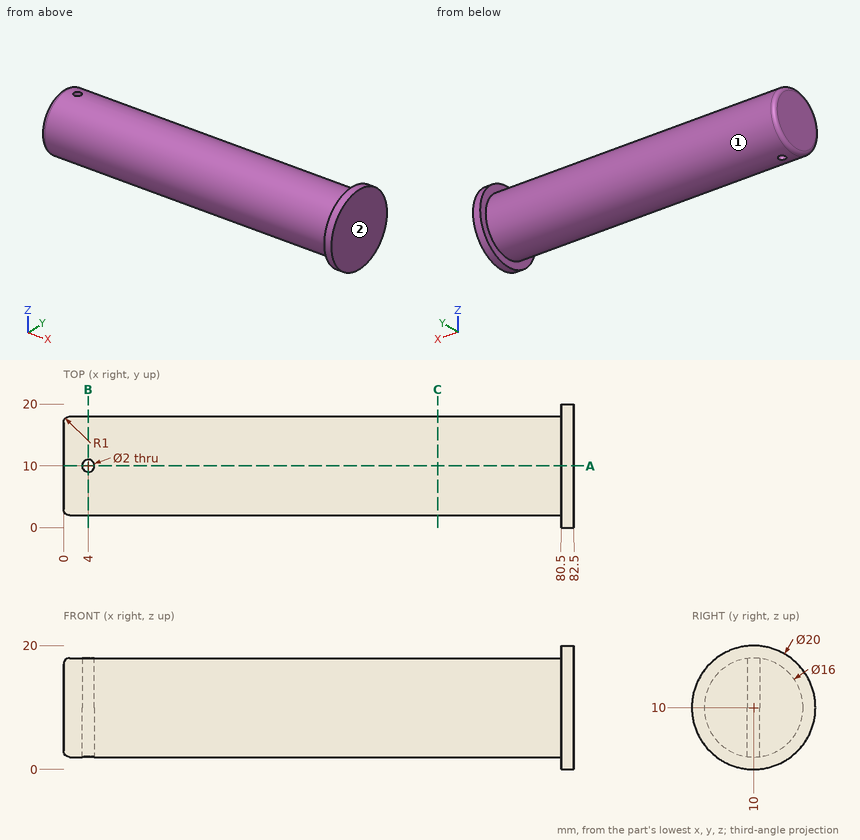
The figure shows three views and two pictorial views of one solid part (mm, origin at its lowest corner). Answer the questions. A direction names the side the tool comes from. Coordinates: 2 decimals unless noted, no trailing zeros. Loops run counter-clockwise (first coordinate to the right, second up) from the corner with the lowest first, then second, coordinate; pieces in that order, holes last. Notation, with made-up numbers: (-39.5, -13) -> (-15.5, -13) arc R22 cw to (-15.5, 7) -> close; hole circle Ø7 at (34, 58). An arc over 180 degrees is marked (long way). Write item = value, one per line. Start each with the question number.
1) A tool of negligible diameter and unlimited length cuts with its end or side. For the marked faces 1 and 2, from which of +Z, -Z, +X, -X, +Y, -Y can it reach the whole face along a straight path? Write none if from no direction.
2) Given pin 1 Ø4 at (x, z) = (12, 12.5) entering from +Y; pin 2 Ø1.5 at (y, z) = (17, 4) entering from -X; pin 3 Ø2.5 at (x, y) = (4, 10) entering from -Z, each flat-ended and moving along its own axis, determine where each tip first touches the part or whether it passes through.
3) A cutting plane is placed at C-C (x = 60.5). Give the vertices of the cut face in (y, z).
4) Straight lines are drawn through the part: line 1 (X direction, y = 10, z = 7); line 2 (Y direction, x = 4, z = 15.5); line 3 (Y direction, x = 4, z = 5.75). For each, find the intervals that lie inside material, in ascending order. Write a range as from..to.
5) A cutting plane is placed at A-A (y = 10). Give the vertices of the cut face in (x, z), then the cut area to 3 significant figures.
6) A cutting plane is placed at B-B (x = 4). Give the vertices of the cut face in (y, z), then the cut area to 3 significant figures.
Responses:
q1.face_1 = -X
q1.face_2 = +Z, -Z, +X, +Y, -Y
q2.pin_1 = 17.98
q2.pin_2 = 80.5
q2.pin_3 = 2
q3.outline = circle Ø16 at (10, 10)
q4.line_1 = 0..3, 5..82.5
q4.line_2 = 4.19..9, 11..15.81
q4.line_3 = 3.22..9, 11..16.78
q5.outline = (0, 3) arc R1 ccw to (1, 2) -> (3, 2) -> (3, 18) -> (1, 18) arc R1 ccw to (0, 17) -> close; (5, 2) -> (80.5, 2) -> (80.5, 0) -> (82.5, 0) -> (82.5, 20) -> (80.5, 20) -> (80.5, 18) -> (5, 18) -> close
q5.area = 1,300 mm²
q6.outline = (9, 2.06) -> (9, 17.94) arc R8 ccw to start; (11, 2.06) arc R8 ccw to (11, 17.94) -> close
q6.area = 169 mm²
